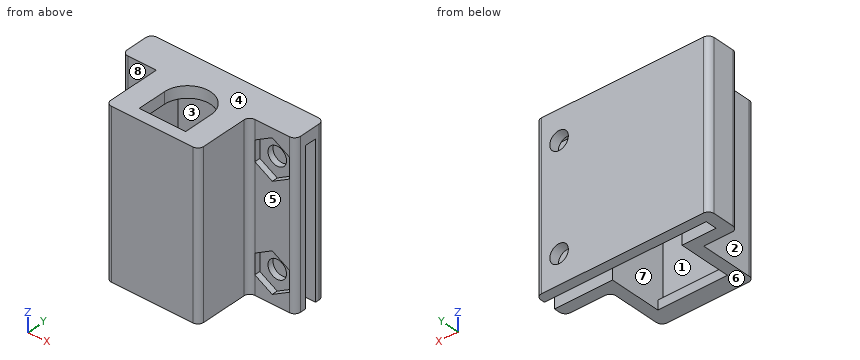
```python
from build123d import *

# Parameters (mm, degrees)
EXTRUDE_1_DEPTH          = 2
EXTRUDE_2_DEPTH          = 26
SKETCH_6_W               = 12
SKETCH_6_H               = 1
EXTRUDE_3_DEPTH          = 1.6
CUT_EXTRUDE_1_DEPTH      = 11
CUT_EXTRUDE_1_DEPTH_BACK = 1
SKETCH_5_R               = 1.6
CUT_EXTRUDE_2_DEPTH      = 5.7


with BuildPart() as part:
    # 草图1 → 凸台-拉伸1 (new body)
    with BuildSketch(Plane.XY):
        with BuildLine():
            ThreePointArc((8, 2), (8.292893219, 2.707106781), (9, 3))
            Line((9, 3), (15, 3))
            ThreePointArc((15, 3), (15.707106781, 3.292893219), (16, 4))
            Line((16, 4), (16, 7.7))
            ThreePointArc((16, 7.7), (15.707106781, 8.407106781), (15, 8.7))
            Line((15, 8.7), (-12.875, 8.7))
            ThreePointArc((-12.875, 8.7), (-13.582106781, 8.407106781), (-13.875, 7.7))
            Line((-13.875, 7.7), (-13.875, 4))
            ThreePointArc((-13.875, 4), (-13.582106781, 3.292893219), (-12.875, 3))
            Line((-12.875, 3), (-8, 3))
            Line((-8, 3), (-8, -6))
            ThreePointArc((-8, -6), (-7.707106781, -6.707106781), (-7, -7))
            Line((-7, -7), (7, -7))
            ThreePointArc((7, -7), (7.707106781, -6.707106781), (8, -6))
            Line((8, -6), (8, 2))
        make_face()
        with BuildLine():
            Line((4, -5), (-4, -5))
            Line((-4, -5), (-4, 0))
            ThreePointArc((-4, 0), (0, 4), (4, 0))
            Line((4, 0), (4, -5))
        make_face(mode=Mode.SUBTRACT)
    extrude(amount=EXTRUDE_1_DEPTH)

    # 草图2 → 凸台-拉伸2 (add)
    with BuildSketch(Plane(origin=(0, 0, 0), x_dir=(-1, 0, 0), z_dir=(0, 0, -1))):
        with BuildLine():
            Line((6, -4), (6, -5))
            Line((6, -5), (5, -5))
            Line((5, -5), (-5, -5))
            Line((-5, -5), (-6, -5))
            Line((-6, -5), (-6, -4))
            Line((-6, -4), (-6, 4))
            Line((-6, 4), (-6, 5))
            Line((-6, 5), (-16, 5))
            Line((-16, 5), (-16, 4))
            ThreePointArc((-16, 4), (-15.707106781, 3.292893219), (-15, 3))
            Line((-15, 3), (-9, 3))
            ThreePointArc((-9, 3), (-8.292893219, 2.707106781), (-8, 2))
            Line((-8, 2), (-8, -6))
            ThreePointArc((-8, -6), (-7.707106781, -6.707106781), (-7, -7))
            Line((-7, -7), (7, -7))
            ThreePointArc((7, -7), (7.707106781, -6.707106781), (8, -6))
            Line((8, -6), (8, 3))
            Line((8, 3), (12.875, 3))
            ThreePointArc((12.875, 3), (13.582106781, 3.292893219), (13.875, 4))
            Line((13.875, 4), (13.875, 7.7))
            ThreePointArc((13.875, 7.7), (13.582106781, 8.407106781), (12.875, 8.7))
            Line((12.875, 8.7), (-15, 8.7))
            ThreePointArc((-15, 8.7), (-15.707106781, 8.407106781), (-16, 7.7))
            Line((-16, 7.7), (-16, 7))
            Line((-16, 7), (11.875, 7))
            Line((11.875, 7), (11.875, 5))
            Line((11.875, 5), (6, 5))
            Line((6, 5), (6, 4))
            Line((6, 4), (6, -4))
        make_face()
    extrude(amount=EXTRUDE_2_DEPTH)

    # 草图6 → 凸台-拉伸3 (add)
    with BuildSketch(Plane(origin=(0, 0, -26), x_dir=(-1, 0, 0), z_dir=(0, 0, -1))):
        with Locations((0, -4.5)):
            Rectangle(SKETCH_6_W, SKETCH_6_H)
    extrude(amount=-EXTRUDE_3_DEPTH)

    # 草图4 → 切除-拉伸1 (cut, two sides)
    with BuildSketch(Plane.XZ.offset(-3)) as cut_extrude_1_sk:
        Polygon((15, -19.267949192), (12, -17.535898385), (9, -19.267949192), (9, -22.732050808), (12, -24.464101615), (15, -22.732050808), align=None)
        Polygon((9, -1.267949192), (9, -4.732050808), (12, -6.464101615), (15, -4.732050808), (15, -1.267949192), (12, 0.464101615), align=None)
    extrude(amount=CUT_EXTRUDE_1_DEPTH, mode=Mode.SUBTRACT)
    extrude(cut_extrude_1_sk.sketch, amount=-CUT_EXTRUDE_1_DEPTH_BACK, mode=Mode.SUBTRACT)

    # 草图5 → 切除-拉伸2 (cut, through all)
    with BuildSketch(Plane.XZ.offset(-4)):
        with Locations((12, -21)):
            Circle(SKETCH_5_R)
        with Locations((12, -3)):
            Circle(SKETCH_5_R)
    extrude(amount=-CUT_EXTRUDE_2_DEPTH, mode=Mode.SUBTRACT)


solid = part.part
```
Part model, mm, in its own coordinate system. Face numbers are marked on the shaded views. A direction names the side the tool comes from. Coordinates: 2 decimals unless noted, no trailing zeros. Write each loop counter-clockwise with the first axis right and the second up, starting at its lowest first coordinate (ties: lowest second). Pieces come first, ordered by that corner, then holes.
Item 1: Slice it at D-D (z = -12). Write the cut outline in (x, y) (3 decimals), and give its area (3 significant figures).
Item 2: Slice it at A-A (z = -3). Count the separate pieces of the cut face and the enclosed holes in it, and give its area (3 significant figures).
Item 3: Mould opens along Y. For the marked faces 6, 7 and 8 say: released by +Y, released by -Y, zero draft, split by the parting line, or undercut.
Item 4: Pin check, flat tips, straight feed: pin 1 (6.5 mm diameter, centred on x = 13, z = -4, fed in from -Y); pin 2 (3 mm diameter, centred on y = -2, z = -11.5, fed in from +X); pin 3 (1.6 mm diameter, centred on y = -3, z = 1, fed in from -X). Stop position of each tip, or through.
Item 5: Slice it at B-B (x = 0). Write the cut outline in (y, z).
Item 6: Slice it at C-C (y = 2.5). Write the cut outline in (x, z), and give its area (3 significant figures).
Item 7: Which spindle directions (+Z, -Z, +X, -X, +Y, -Y) get a long thin tool onto all of the face, cutting with end or side? Do the marked faces 1, 2, 3, 4 and 5. Say none if no direction does.
Item 8: Probe line 1 (Z direction, x = 12, y = 4.4); line 2 (Y direction, x = 14.5, z = -10.75); line 3 (X direction, y = -4, z = -13.5). List the from-to ranges inside material, lowest first.
Results found:
1. outline: (-13.875, 4) arc R1 ccw to (-12.875, 3) - (-8, 3) - (-8, -6) arc R1 ccw to (-7, -7) - (7, -7) arc R1 ccw to (8, -6) - (8, 2) arc R1 cw to (9, 3) - (15, 3) arc R1 ccw to (16, 4) - (16, 5) - (6, 5) - (6, -5) - (-6, -5) - (-6, 5) - (-11.875, 5) - (-11.875, 7) - (16, 7) - (16, 7.7) arc R1 ccw to (15, 8.7) - (-12.875, 8.7) arc R1 ccw to (-13.875, 7.7) - close
1. area: 153 mm2
2. separate pieces: 3
2. enclosed holes: 0
2. area: 139 mm2
3. face 6: zero draft
3. face 7: undercut
3. face 8: released by -Y
4. pin 1: stops at y = 3
4. pin 2: stops at x = 8
4. pin 3: stops at x = -8
5. outline: (-7, -26) - (-4, -26) - (-4, -24.4) - (-5, -24.4) - (-5, 2) - (-7, 2) - close; (4, 0) - (7, 0) - (7, -26) - (8.7, -26) - (8.7, 2) - (4, 2) - close
6. outline: (-8, -26) - (-6, -26) - (-6, 0) - (-3.12, 0) - (-3.12, 2) - (-8, 2) - close; (3.12, 0) - (6, 0) - (6, -26) - (8.13, -26) - (8.13, 2) - (3.12, 2) - close
6. area: 127 mm2
7. face 1: none
7. face 2: +Z, -Z, -X, -Y
7. face 3: -Z, +X
7. face 4: +Z, +X, -X, +Y, -Y
7. face 5: +Z, -Z, +X, -Y
8. line 1: z = -26 to -22.6, -19.4 to -4.6, -1.4 to 2
8. line 2: y = 3 to 5, 7 to 8.7
8. line 3: x = -8 to -6, 6 to 8
